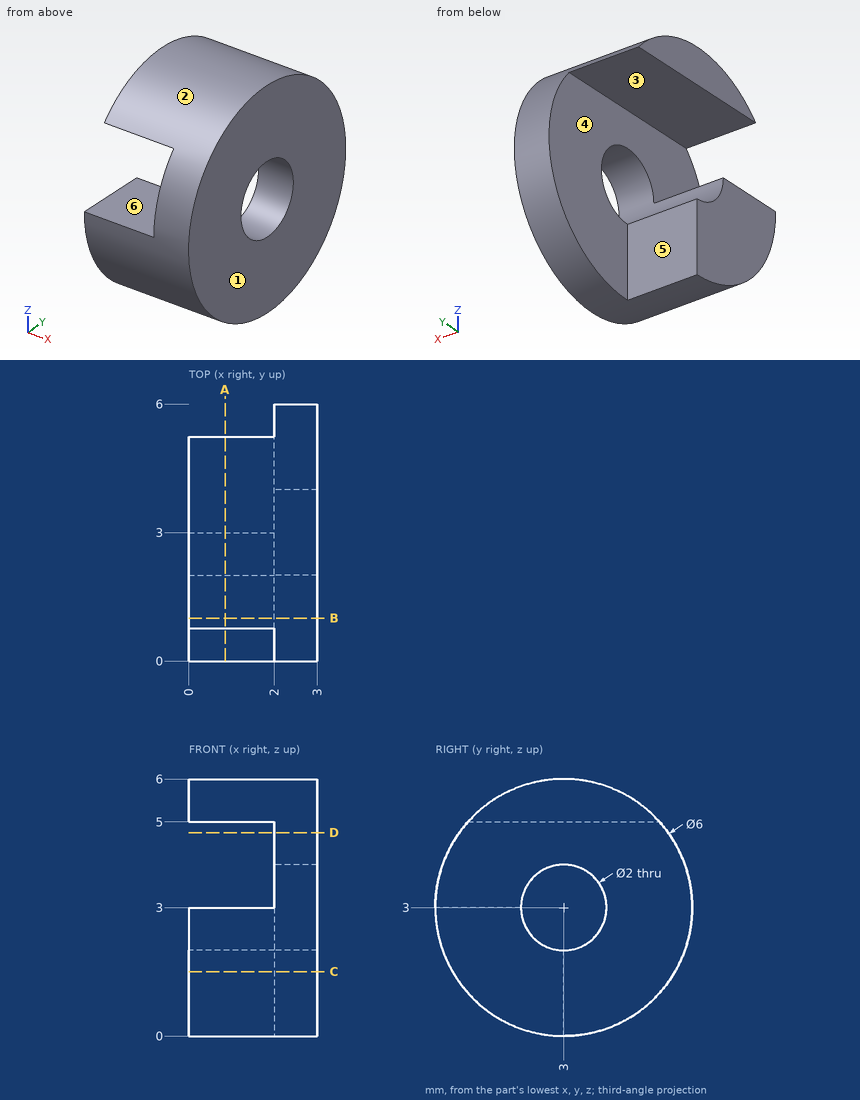
Design review of the part shown in the three views and the two pictorial views. Dimensions are in mm from the part's minimum x, y and z. A direction names the side the tool comes from. Coordinates: 2 decimals unless noted, no trailing zeros. Order: outer loops, then holes, each group sorted by start corner. A loop starts at its lowest first (then second) coordinate and runs counter-clockwise, first axis right, second up.
Item 1: For line 1 (X direction, y = 5.5, z = 2.5); line 2 (Z direction, x = 1.85, y = 2.5); line 3 (Z direction, x = 2.7, y = 1), list the stretches that pass through material, from the lowest coordinate up.
Item 2: The part is to be moulded in two halves that separate along Z. For the marked faces 1, 2 and 3, say which applies: pulls with the +Z half, pulls with the -Z half, needs draft (parallel to the pull), parting line crosses it, or undercut.
Item 3: For the marked faces 4, 5 and 6, list the 3-axis set-ups (+Z, -Z, +X, -X, +Y, -Y) from which the entire face can be reached by the end or side of a thin tool; tool diameter is ignored.
Item 4: For pin 1 Ø1.6 at (x, z) = (1, 1) entering from +Y; pin 2 Ø1.5 at (y, z) = (4, 1.5) entering from -X; pin 3 Ø1 at (x, z) = (0.5, 1) entering from -Y, all flat-tipped, find the tip position at first contact; note any pin that passes through.
Item 5: Take a section at B-B, the plane y = 1. Write out the cut boundary in (x, z).
Item 6: Take a section at A-A, the plane x = 0.85. Write out the cut boundary in (y, z).
Item 7: Take a section at C-C, the plane z = 1.5. Write out the cut boundary in (x, y), then the cut area to 3 significant figures.
Item 8: Take a section at D-D, the plane z = 4.75. Write out the cut boundary in (x, y).
The answers:
1. line 1: x = 2 to 3
1. line 2: z = 0.04 to 2.13, 5 to 5.96
1. line 3: z = 0.76 to 5.24
2. face 1: needs draft
2. face 2: parting line crosses it
2. face 3: undercut
3. face 4: -X, +Y
3. face 5: -Z, -X, +Y
3. face 6: -X, +Y, -Y
4. pin 1: stops at y = 3
4. pin 2: stops at x = 2
4. pin 3: stops at y = 0.4
5. outline: (0, 0.76) - (3, 0.76) - (3, 5.24) - (0, 5.24) - (0, 5) - (2, 5) - (2, 3) - (0, 3) - close
6. outline: (0, 3) arc R3 ccw to (3, 0) - (3, 2) arc R1 cw to (2, 3) - close; (0.76, 5) - (5.24, 5) arc R3 ccw to start
7. outline: (0, 0.4) - (3, 0.4) - (3, 5.6) - (2, 5.6) - (2, 3) - (0, 3) - close
7. area: 10.4 mm2
8. outline: (2, 0.56) - (3, 0.56) - (3, 5.44) - (2, 5.44) - close
